```python
from build123d import *

# Parameters (mm, degrees)
F0_W     = 97.5
F0_H     = 24
F0_W_2   = 68
F0_H_2   = 18.6
F1_DEPTH = 51
F2_DEPTH = 2
F3_W     = 16
F3_H     = 12
F4_DEPTH = 25
F5_R     = 1


with BuildPart() as f1:
    # F0 (on Top) → F1 (new body)
    with BuildSketch(Plane.XY):
        with Locations((7.836403, -3.65245)):
            Rectangle(F0_W, F0_H)
        with Locations((7.836403, -3.65245)):
            Rectangle(F0_W_2, F0_H_2, mode=Mode.SUBTRACT)
    extrude(amount=F1_DEPTH)

    # F0 (on Top) → F2 (join)
    with BuildSketch(Plane.XY):
        with Locations((7.836403, -3.65245)):
            Rectangle(F0_W_2, F0_H_2)
    extrude(amount=F2_DEPTH)

    # F3 (on face) → F4 (cut)
    with BuildSketch(Plane(origin=(-40.913597, 0, 0), x_dir=(0, -1, 0), z_dir=(-1, 0, 0))):
        with Locations((3.65245, 20)):
            Rectangle(F3_W, F3_H)
    extrude(amount=-F4_DEPTH, mode=Mode.SUBTRACT)

    # F5
    f5_edges = [f1.edges().sort_by_distance(p)[0] for p in [
        (-40.913597, -15.65245, 25.5),
        (-40.913597, 8.34755, 25.5),
        (56.586403, -15.65245, 25.5),
        (56.586403, 8.34755, 25.5),
        (41.836403, 5.64755, 26.5),
        (41.836403, -12.95245, 26.5),
        (-26.163597, 5.64755, 26.5),
        (-26.163597, -12.95245, 26.5),
    ]]
    fillet(f5_edges, radius=F5_R)


solid = f1.part
```
Here's how the part is built. I have some questions about the finished solid (model axes, mm). A direction names the side the tool comes from. Give positions to 0.01 mm unless a question says otherwise; leave off trailing zeros. Write each loop counter-clockwise with the first axis right and the second up, starting at its lowest first coordinate (ties: lowest second). Pieces come first, ordered by that corner, then holes. Notation, with made-up numbers: (41, 3) -> (84, 3) arc R25 ccw to (84, 35) -> close; hole circle Ø2 at (-15, 38). An arc over 180 degrees is marked (long way). Use one line per item in the form item = value.
1) Suppose I cut it at B-B (z = 36.5). Please give me the cut outline in (x, y).
Verdict:
outline = (-40.91, -14.65) arc R1 ccw to (-39.91, -15.65) -> (55.59, -15.65) arc R1 ccw to (56.59, -14.65) -> (56.59, 7.35) arc R1 ccw to (55.59, 8.35) -> (-39.91, 8.35) arc R1 ccw to (-40.91, 7.35) -> close; hole (-26.16, -11.95) arc R1 ccw to (-25.16, -12.95) -> (40.84, -12.95) arc R1 ccw to (41.84, -11.95) -> (41.84, 4.65) arc R1 ccw to (40.84, 5.65) -> (-25.16, 5.65) arc R1 ccw to (-26.16, 4.65) -> close
2) We'd pull the mould along X, two halves only. Please class faces 4 (the face through (7, 5.648, 26)), 5 (the face through (56.586, -4, 25)), 6 (the face through (-40.914, -4, 31)): +X half, -X half, draft (parallel to the pull), parting line (faces both ways), or undercut.
Verdict:
face_4 = undercut
face_5 = +X half
face_6 = -X half
3) Suppose I cut it at A-A (y = 2). Please give me the cut outline in (x, z), and give its area (3 significant figures).
Verdict:
outline = (-40.91, 0) -> (56.59, 0) -> (56.59, 51) -> (41.84, 51) -> (41.84, 2) -> (-26.16, 2) -> (-26.16, 14) -> (-40.91, 14) -> close; (-40.91, 26) -> (-26.16, 26) -> (-26.16, 51) -> (-40.91, 51) -> close
area = 1,460 mm2
4) Suppose I cut it at C-C (x = -5). Please give me the cut outline in (y, z), and give its area (3 significant figures).
Verdict:
outline = (-15.65, 0) -> (8.35, 0) -> (8.35, 51) -> (5.65, 51) -> (5.65, 2) -> (-12.95, 2) -> (-12.95, 51) -> (-15.65, 51) -> close
area = 313 mm2
5) If I drill on L1, parallel to Y at x = 16.5, z = 11; L2, parallel to X at y = 2, z = 38; L3, parallel to Y at x = 41, z = 45, over which ranges is the centre line in solid material (lowest first)? Write a range as [from, to].
Verdict:
L1 = [-15.65, -12.95], [5.65, 8.35]
L2 = [-40.91, -26.16], [41.84, 56.59]
L3 = [-15.65, -12.94], [5.63, 8.35]
6) I'm going to push a flat-ended pin straight in: pin 1 (5.5 mm diameter, centred on x = 1.5, y = -8, fed in from +Z). Where does the tip first touch, or does it pass through?
Verdict:
pin_1 = 2
7) On a 3-axis mill with a long thin cutter (end or side, diameter ignored), from which of +Z, -Z, +X, -X, +Y, -Y can I reach the whole of each face in a straight line? I mean faces 1 (the face through (-34, -4, 26)), 2 (the face through (7, -12.952, 26)), 3 (the face through (7, 8.348, 25)). Say none if no direction works.
Verdict:
face_1 = -X
face_2 = +Z
face_3 = +Z, -Z, +X, -X, +Y
